Geometry: see drawing. Coordinates: mm, zero at the bounding-box minimum. Coordinates: 2 decimals unless noted, no trailing zeros. Write each loop counter-clockwise with the first axis right and the second up, starting at its lowest first coordinate (ties: lowest second). Pieces come first, ordered by that corner, then holes.
1) Section query D-D (x = 273.5). Output: boundary loops of the cut face in (y, z) (1 decimal), then the cut area to 3 significant figures.
2) Pin query (flat end, axial travel): pin 1 Ø5 at (y, z) = (175, 17) entering from -X (1 decimal); pin 2 Ø1.5 at (x, z) = (209.5, 20) entering from -Y; pin 3 Ø10 at (x, z) = (717.5, 18.5) entering from +Y (1 decimal). Return the tip coordinate at first contact, or that it passes through.
3) Section query A-A (y = 235). Output: boundary loops of the cut face in (x, z).
4) Section query C-C (y = 347). Output: boundary loops of the cut face in (x, z) (1 decimal), then the cut area to 3 significant figures.
5) Line query: L1, parallel to X at y = 151.5, z = 22.75 (1 decimal); L2, parallel to Y at x = 741, z = 16 (1 decimal); L3, parallel to Y at x = 136, z = 5 (1 decimal). Output: solid intervals per line, ascending.
6) Section query B-B (z = 18.75). State how many separate pieces and enclosed holes the cut face has, then the cut area to 3 significant figures.
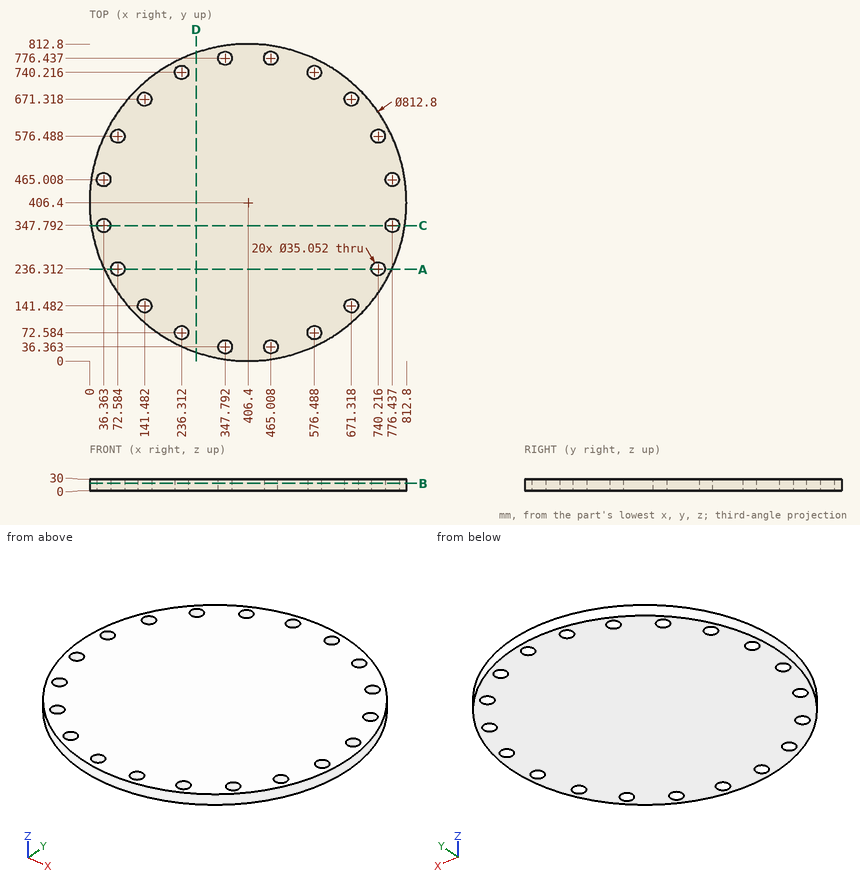
Answer:
1. outline: (22.3, 0) - (790.5, 0) - (790.5, 30) - (22.3, 30) - close
1. area: 23,000 mm2
2. pin 1: stops at x = 70.6
2. pin 2: stops at y = 50.47
2. pin 3: stops at y = 673.7
3. outline: (37.91, 0) - (55.11, 0) - (55.11, 30) - (37.91, 30) - close; (90.06, 0) - (722.74, 0) - (722.74, 30) - (90.06, 30) - close; (757.69, 0) - (774.89, 0) - (774.89, 30) - (757.69, 30) - close
4. outline: (4.4, 0) - (18.9, 0) - (18.9, 30) - (4.4, 30) - close; (53.9, 0) - (758.9, 0) - (758.9, 30) - (53.9, 30) - close; (793.9, 0) - (808.4, 0) - (808.4, 30) - (793.9, 30) - close
4. area: 22,000 mm2
5. L1: x = 89.9 to 127.1, 155.9 to 656.9, 685.7 to 722.9
5. L2: y = 175.7 to 218.8, 253.8 to 559, 594 to 637.1
5. L3: y = 103 to 124.8, 158.1 to 654.7, 688 to 709.8
6. separate pieces: 1
6. enclosed holes: 20
6. area: 500,000 mm2
